```python
from build123d import *

# Parameters (mm, degrees)
BOSS_EXTRUDE1_DEPTH = 0.8
BOSS_EXTRUDE2_DEPTH = 0.8


with BuildPart() as part:
    # Sketch1 → Boss-Extrude1 (new body)
    with BuildSketch(Plane.XY):
        Polygon((-1.25, 2.5), (1.25, 2.5), (1.75, 2), (2.5, 2), (2.5, -2), (1.75, -2), (1.25, -2.5), (-1.25, -2.5), (-1.75, -2), (-2.5, -2), (-2.5, 2), (-1.75, 2), align=None)
    extrude(amount=BOSS_EXTRUDE1_DEPTH)

    # Sketch2 → Revolve1 (revolve)
    with BuildSketch(Plane(origin=(0, 0, 0), x_dir=(1, 0, 0), z_dir=(0, 1, 0)), mode=Mode.PRIVATE) as revolve1_sk:
        Polygon((0, -0.8), (0, -3.2), (2.3, -3.2), (2, -2.787085424), (2, -1.212914576), (2.3, -0.8), align=None)
    revolve(revolve1_sk.sketch.rotate(Axis((0, 0, 0.8), (0, 0, 1)), 180), axis=Axis((0, 0, 0.8), (0, 0, 1)))

    # Sketch3 → Boss-Extrude2 (add)
    with BuildSketch(Plane.XY.offset(3.2)):
        Polygon((-1.25, 2.5), (1.25, 2.5), (2.4, 1.35), (2.4, -1.35), (1.25, -2.5), (-1.25, -2.5), (-2.4, -1.35), (-2.4, 1.35), align=None)
    extrude(amount=BOSS_EXTRUDE2_DEPTH)


solid = part.part
```
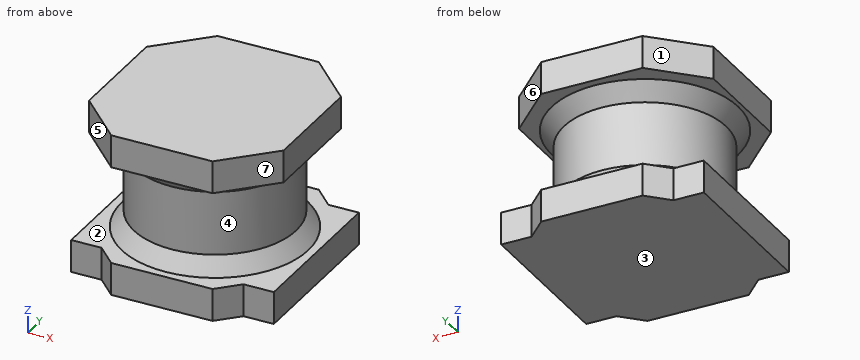
Could you check a few things on this model? Use its own coordinates, in mm. Face numbers are marked on the shaded views. A direction names the side the tool comes from. Coordinates: 2 decimals unless noted, no trailing zeros. Order: outer loops, then holes, each group sorted by start corner. A loop starts at its lowest first (then second) coordinate and runs counter-clockwise, first axis right, second up. Notation, with made-up numbers: M 51,17 L 72,17 A18 cw 72,39 Z; hole C -17.5,71.25 d4. An arc over 180 degrees is marked long. Use one line per item in the form item = value. Start each with the question number.
1. Suppose I cut it at C-C on z = 1.65. Write out the boundary of the cut face in (x, y), then the cut area to 3 significant figures.
2. We'd pull the mould along Z, two halves only. Please class the marked faces 1, 2 and 3: +Z half, -Z half, draft (parallel to the pull), parting line (faces both ways), or undercut.
3. On a 3-axis mill with a long thin cutter (end or side, diameter ignored), from which of +Z, -Z, +X, -X, +Y, -Y can I reach the whole of each face in a straight line? I mean the marked faces 4, 5, 6 and 7. Say none if no direction works.
4. Suppose I cut it at A-A on x = 0. Write out the boundary of the cut face in (y, z).
5. For pin 1 (2 mm diameter, centred on y = -1, z = 3, fed in from -X); pin 2 (1 mm diameter, centred on x = 1.5, y = -1.5, fed in from -Z); pin 3 (1 mm diameter, centred on x = -1.5, z = 1.5, fed in from +Y); pin 4 (0.6 mm diameter, centred on x = 2, z = 0, fed in from -Y), each with a flat end and sliding along its axis, tell me the tip position at first contact or that it passes through.
6. Please list where these lines run through material, in increasing order: line 1 (Z direction, x = -2, y = -1.3); line 2 (X direction, y = 1.25, z = 3.6); line 3 (Z direction, x = 1.6, y = -1.6).
7. Suppose I cut it at B-B on y = 0. Write out the boundary of the cut face in (x, z), then the cut area to 3 significant figures.
Geometry says:
q1.outline = C 0,0 d4
q1.area = 12.6 mm^2
q2.face_1 = draft
q2.face_2 = undercut
q2.face_3 = -Z half
q3.face_4 = none
q3.face_5 = +Z, -X, -Y
q3.face_6 = +Z, +X, +Y
q3.face_7 = +Z, +X, -Y
q4.outline = M -2.5,0 L 2.5,0 L 2.5,0.8 L 2.3,0.8 L 2,1.21 L 2,2.79 L 2.3,3.2 L 2.5,3.2 L 2.5,4 L -2.5,4 L -2.5,3.2 L -2.3,3.2 L -2,2.79 L -2,1.21 L -2.3,0.8 L -2.5,0.8 Z
q5.pin_1 = -2.4
q5.pin_2 = 0
q5.pin_3 = 1.73
q5.pin_4 = -2.05
q6.line_1 = 0 to 0.8, 3.2 to 4
q6.line_2 = -2.4 to 2.4
q6.line_3 = 0 to 0.85, 3.15 to 4
q7.outline = M -2.5,0 L 2.5,0 L 2.5,0.8 L 2.3,0.8 L 2,1.21 L 2,2.79 L 2.3,3.2 L 2.4,3.2 L 2.4,4 L -2.4,4 L -2.4,3.2 L -2.3,3.2 L -2,2.79 L -2,1.21 L -2.3,0.8 L -2.5,0.8 Z
q7.area = 17.7 mm^2
